```python
from build123d import *

# Parameters (mm, degrees)
SKETCH1_W           = 120
SKETCH1_H           = 55
BOSS_EXTRUDE1_DEPTH = 5
SKETCH2_W           = 120
SKETCH2_H           = 7.5
BOSS_EXTRUDE2_DEPTH = 20
SKETCH3_W           = 120
SKETCH3_H           = 2.5
BOSS_EXTRUDE4_DEPTH = 20
BOSS_EXTRUDE5_DEPTH = 190
SKETCH9_W           = 310
SKETCH9_H           = 25
BOSS_EXTRUDE6_DEPTH = 70
SKETCH14_R          = 5.5
CUT_EXTRUDE5_DEPTH  = 153
SKETCH15_W          = 125
SKETCH15_H          = 25
CUT_EXTRUDE6_DEPTH  = 190
SKETCH16_W          = 120
SKETCH16_H          = 125
BOSS_EXTRUDE8_DEPTH = 10
SKETCH17_W          = 120
SKETCH17_H          = 125
CUT_EXTRUDE7_DEPTH  = 18
CUT_EXTRUDE8_START  = -18
SKETCH18_R          = 5.5
CUT_EXTRUDE8_DEPTH  = 18


with BuildPart() as part:
    # Sketch1 → Boss-Extrude1 (new body)
    with BuildSketch(Plane(origin=(0, 0, 0), x_dir=(1, 0, 0), z_dir=(0, 1, 0))):
        Rectangle(SKETCH1_W, SKETCH1_H)
    extrude(amount=BOSS_EXTRUDE1_DEPTH)

    # Sketch2 → Boss-Extrude2 (add)
    with BuildSketch(Plane(origin=(0, 5, 0), x_dir=(1, 0, 0), z_dir=(0, 1, 0))):
        with Locations((0, -23.75)):
            Rectangle(SKETCH2_W, SKETCH2_H)
    extrude(amount=BOSS_EXTRUDE2_DEPTH)

    # Sketch3 → Boss-Extrude4 (add)
    with BuildSketch(Plane(origin=(0, 5, 0), x_dir=(1, 0, 0), z_dir=(0, 1, 0))):
        with Locations((0, 26.25)):
            Rectangle(SKETCH3_W, SKETCH3_H)
    extrude(amount=BOSS_EXTRUDE4_DEPTH)

    # Sketch8 → Boss-Extrude5 (add)
    with BuildSketch(Plane.ZY.offset(60)):
        Polygon((-27.5, 0), (-27.5, 25), (-25, 25), (-25, 5), (20, 5), (20, 25), (27.5, 25), (27.5, 0), align=None)
    extrude(amount=BOSS_EXTRUDE5_DEPTH)

    # Sketch9 → Boss-Extrude6 (add)
    with BuildSketch(Plane(origin=(0, 0, -27.5), x_dir=(-1, 0, 0), z_dir=(0, 0, -1))):
        with Locations((95, 12.5)):
            Rectangle(SKETCH9_W, SKETCH9_H)
    extrude(amount=BOSS_EXTRUDE6_DEPTH)

    # Sketch14 → Cut-Extrude5 (cut)
    with BuildSketch(Plane(origin=(0, 0, 0), x_dir=(-1, 0, 0), z_dir=(0, -1, 0))):
        with Locations(Location((225.445279058, 7.255161462, 0), (0, 0, 90))):
            Circle(SKETCH14_R)
        with Locations(Location((175.445279058, 7.255161462, 0), (0, 0, 90))):
            Circle(SKETCH14_R)
        with Locations(Location((225.445279058, 57.255161462, 0), (0, 0, 90))):
            Circle(SKETCH14_R)
        with Locations(Location((148.0182107, 48.5, 0), (0, 0, 90))):
            Circle(SKETCH14_R)
        with Locations(Location((183.240850763, 83.987541856, 0), (0, 0, 90))):
            Circle(SKETCH14_R)
    extrude(amount=-CUT_EXTRUDE5_DEPTH, mode=Mode.SUBTRACT)

    # Sketch15 → Cut-Extrude6 (cut)
    with BuildSketch(Plane(origin=(60, 0, 0), x_dir=(0, 0, -1), z_dir=(1, 0, 0))):
        with Locations((35, 12.5)):
            Rectangle(SKETCH15_W, SKETCH15_H)
    extrude(amount=-CUT_EXTRUDE6_DEPTH, mode=Mode.SUBTRACT)

    # Sketch16 → Boss-Extrude8 (add)
    with BuildSketch(Plane(origin=(0, 0, 0), x_dir=(-1, 0, 0), z_dir=(0, -1, 0))):
        with Locations((190, 35)):
            Rectangle(SKETCH16_W, SKETCH16_H)
    extrude(amount=BOSS_EXTRUDE8_DEPTH)

    # Sketch17 → Cut-Extrude7 (cut)
    with BuildSketch(Plane(origin=(0, 25, 0), x_dir=(1, 0, 0), z_dir=(0, 1, 0))):
        with Locations((-190, 35)):
            Rectangle(SKETCH17_W, SKETCH17_H)
    extrude(amount=-CUT_EXTRUDE7_DEPTH, mode=Mode.SUBTRACT)

    # Sketch18 → Cut-Extrude8 (cut)
    with BuildSketch(Plane(origin=(0, 7, 0), x_dir=(1, 0, 0), z_dir=(0, 1, 0)).offset(CUT_EXTRUDE8_START)):
        with Locations(Location((-148.0182107, 48.5, 0), (0, 0, 270))):
            Circle(SKETCH18_R)
    extrude(amount=CUT_EXTRUDE8_DEPTH, mode=Mode.SUBTRACT)


solid = part.part
```
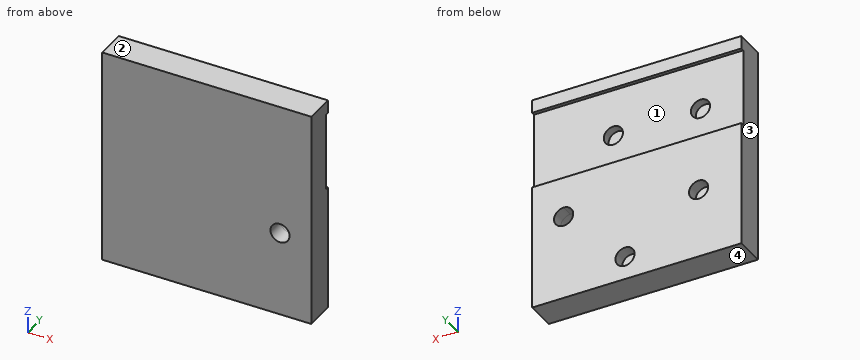
Work out the finished part from the listing and answer in its coordinate system (mm). Face numbers are marked on the shaded views. Give positions to 0.01 mm unless a question says otherwise; leave off trailing zeros. Order: outer loops, then holes, each group sorted by start corner. A loop starts at its lowest first (then second) coordinate and runs counter-clockwise, first axis right, second up. Notation, with made-up numbers: (19.25, -12) -> (73.25, -12) arc R21 ccw to (73.25, -1) -> close; hole circle Ø9 at (77, -22). An arc over 180 degrees is marked (long way). Answer as CSV lines item,"result". Start each with the question number.
(1) Section C-C, the plane x = -161.5 is taken. Write down the section's boundary in (y, z).
(2) Section D-D, the plane z = 18 is taken. Write down the section's boundary in (x, y).
(3) For a pull along Z with two mould halves and no side action, classify the marked faces 1, 2, 3 and 4 as released by +Z, released by -Z, zero draft, split by the parting line, or undercut.
(4) Consider line 1 along Y through (x, z) = (-135.5, -18); line 2 along X through (y, z) = (5, -44); line 3 along X through (y, z) = (-7.25, -51). Determine where each line is inside the solid, lowest interval first.
(5) Each of these flat-tipped pins is pushed along its axis until it touches: pin 1 Ø17.5 at (x, z) = (-225.45, -7.26) entering from +Y; pin 2 Ø3.5 at (x, z) = (-181.5, -86) entering from +Y; pin 3 Ø5.5 at (x, z) = (-223, -59.5) entering from +Y; pin 4 Ø6.5 at (x, z) = (-148.02, -48.5) entering from +Y. Where does it stop, or does it pass through?
(6) Section A-A, the plane z = -48.5 is taken. Write down the section's boundary in (x, y), plus the area to 3 significant figures.
(7) Section B-B, the plane y = 3.5 is taken. Write down the section's boundary in (x, z).
Entries:
1,outline,"(-10, -97.5) -> (7, -97.5) -> (7, -25) -> (5, -25) -> (5, 20) -> (7, 20) -> (7, 27.5) -> (-10, 27.5) -> close"
2,outline,"(-250, -10) -> (-130, -10) -> (-130, 5) -> (-250, 5) -> close"
3,face 1,"undercut"
3,face 2,"released by +Z"
3,face 3,"zero draft"
3,face 4,"released by -Z"
4,line 1,"-10 to 5"
4,line 2,"-250 to -151.18, -144.86 to -130"
4,line 3,"-250 to -152.92, -143.12 to -130"
5,pin 1,"y = 5"
5,pin 2,"y = 0"
5,pin 3,"y = 7"
5,pin 4,"through"
6,outline,"(-250, -10) -> (-153.52, -10) -> (-153.52, 7) -> (-250, 7) -> close; (-142.52, -10) -> (-130, -10) -> (-130, 7) -> (-142.52, 7) -> close"
6,area,"1,850 mm²"
7,outline,"(-250, -97.5) -> (-130, -97.5) -> (-130, 27.5) -> (-250, 27.5) -> close; hole circle Ø11 at (-225.45, -57.26); hole circle Ø11 at (-225.45, -7.26); hole circle Ø11 at (-183.24, -83.99); hole circle Ø11 at (-175.45, -7.26); hole circle Ø11 at (-148.02, -48.5)"
